Source: CAD feature listing. Evaluate the final solid. Frame: model axes, mm. Face numbers are marked on the shaded views. Give positions to 0.01 mm unless a question says otherwise; leave off trailing zeros. Order: outer loops, then holes, each group sorted by start corner. A loop starts at its lowest first (then second) coordinate and runs counter-clockwise, first axis right, second up. Notation, with made-up numbers: M 38.5,83 L 55.5,83 A18 cw 55.5,104 Z; hole C 66.5,16 d8. An arc over 180 degrees is marked long. Answer in a Markdown table with one row per item. Add a question column.
(1) Mould query, pull axis Z, two halves, no side actions, for the marked faces 1, 2, 3 and 4. Classes: pulls with the +Z half, pulls with the -Z half, needs draft (parallel to the pull), parting line crosses it, or undercut.
(2) Pin query (flat end, axial travel): P1, Ø6.5, axis at x = -13, z = -5, coming from the +Y side. Return the tip coordinate at first contact, or that it passes through.
(3) Section query D-D, the plane x = -13. Return loops of the section in (y, z).
(4) Material intervals for line 1 along Z through (x, y) = (69.5, -9.5); line 2 along Z through (x, y) = (56.5, -8); line 3 along Z through (x, y) = (75.5, -8), sorted ascending.
(5) Section query A-A, the plane z = -27.25. Return loops of the section in (x, y).
(6) Section query C-C, the plane y = -17.25. Return loops of the section in (x, z), plus the area to 3 significant figures.
(7) Section query B-B, the plane x = 0. Return loops of the section in (y, z).
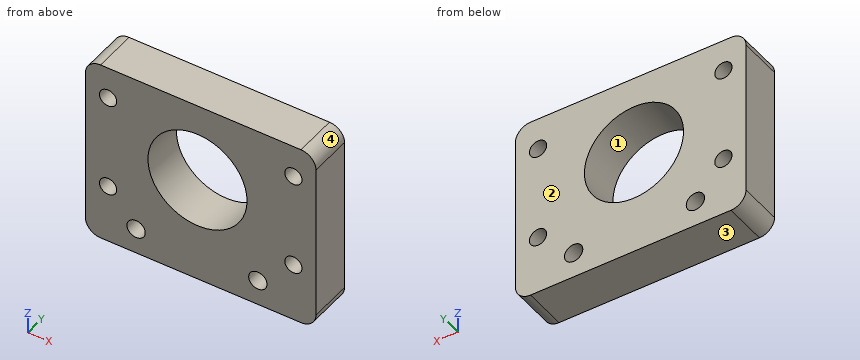
from build123d import *

# Parameters (mm, degrees)
F0_R     = 4.25
F0_R_2   = 4
F0_R_3   = 23
F0_R_4   = 3.35
F1_DEPTH = 20


with BuildPart() as f1:
    # F0 (on Front) → F1 (new body)
    with BuildSketch(Plane.XZ):
        with BuildLine():
            Line((76.5, 10), (-16.5, 10))
            ThreePointArc((-16.5, 10), (-21.449747, 7.949747), (-23.5, 3))
            Line((-23.5, 3), (-23.5, -70))
            ThreePointArc((-23.5, -70), (-21.449747, -74.949747), (-16.5, -77))
            Line((-16.5, -77), (76.5, -77))
            ThreePointArc((76.5, -77), (81.449747, -74.949747), (83.5, -70))
            Line((83.5, -70), (83.5, 3))
            ThreePointArc((83.5, 3), (81.449747, 7.949747), (76.5, 10))
        make_face()
        with Locations((0, -65)):
            Circle(F0_R, mode=Mode.SUBTRACT)
        with Locations((-13, -49.5)):
            Circle(F0_R_2, mode=Mode.SUBTRACT)
        with Locations((56.5, -65)):
            Circle(F0_R, mode=Mode.SUBTRACT)
        with Locations((73, -49.5)):
            Circle(F0_R_2, mode=Mode.SUBTRACT)
        with Locations((28.5, -27.25)):
            Circle(F0_R_3, mode=Mode.SUBTRACT)
        with Locations((-13, -5)):
            Circle(F0_R_2, mode=Mode.SUBTRACT)
        Circle(F0_R_4, mode=Mode.SUBTRACT)
        with Locations((56.5, 0)):
            Circle(F0_R_4, mode=Mode.SUBTRACT)
        with Locations((73, -5)):
            Circle(F0_R_2, mode=Mode.SUBTRACT)
        Circle(F0_R_4)
        with Locations((56.5, 0)):
            Circle(F0_R_4)
    extrude(amount=F1_DEPTH)


solid = f1.part
Values follow:
| question | item | result |
|---|---|---|
| 1 | face 1 | undercut |
| 1 | face 2 | needs draft |
| 1 | face 3 | pulls with the -Z half |
| 1 | face 4 | pulls with the +Z half |
| 2 | P1 | passes through |
| 3 | outline | M -20,-77 L 0,-77 L 0,-53.5 L -20,-53.5 Z; M -20,-45.5 L 0,-45.5 L 0,-9 L -20,-9 Z; M -20,-1 L 0,-1 L 0,10 L -20,10 Z |
| 4 | line 1 | z = -77 to -51.44, -47.56 to -6.94, -3.06 to 10 |
| 4 | line 2 | z = -77 to -69.25, -60.75 to 10 |
| 4 | line 3 | z = -77 to -52.62, -46.38 to -8.12, -1.88 to 10 |
| 5 | outline | M -23.5,-20 L 5.5,-20 L 5.5,0 L -23.5,0 Z; M 51.5,-20 L 83.5,-20 L 83.5,0 L 51.5,0 Z |
| 6 | outline | M -23.5,-70 A7 ccw -16.5,-77 L 76.5,-77 A7 ccw 83.5,-70 L 83.5,3 A7 ccw 76.5,10 L -16.5,10 A7 ccw -23.5,3 Z; hole C -13,-49.5 d8; hole C -13,-5 d8; hole C 0,-65 d8.5; hole C 28.5,-27.25 d46; hole C 56.5,-65 d8.5; hole C 73,-49.5 d8; hole C 73,-5 d8 |
| 6 | area | 7,290 mm² |
| 7 | outline | M -20,-77 L 0,-77 L 0,-69.25 L -20,-69.25 Z; M -20,-60.75 L 0,-60.75 L 0,10 L -20,10 Z |
